```python
from build123d import *

# Parameters (mm, degrees)
SKETCH1_W               = 2.2
SKETCH1_H               = 9.7
SKETCH1_W_2             = 5.7
SKETCH1_H_2             = 3.4
BOSS_EXTRUDE2_DEPTH     = 3
CUT_EXTRUDE2_DEPTH      = 58.983591645
CUT_EXTRUDE2_DEPTH_BACK = 58.983591645
FILLET1_R               = 5
SKETCH4_W               = 20
SKETCH4_H               = 3
BOSS_EXTRUDE3_DEPTH     = 1
SKETCH5_W               = 20
SKETCH5_H               = 1
BOSS_EXTRUDE4_DEPTH     = 10
SKETCH6_W               = 20
SKETCH6_H               = 1.5
BOSS_EXTRUDE5_DEPTH     = 8
SKETCH7_W               = 20
SKETCH7_H               = 3
BOSS_EXTRUDE6_DEPTH     = 1
SKETCH8_W               = 20
SKETCH8_H               = 1
BOSS_EXTRUDE7_DEPTH     = 1.6


with BuildPart() as part:
    # Sketch1 → Boss-Extrude2 (new body)
    with BuildSketch(Plane(origin=(0, 0, 0), x_dir=(1, 0, 0), z_dir=(0, 1, 0))):
        Polygon((0, 15.5), (0, 0), (65, 0), (65, 40), (0, 40), (0, 24.5), (6.46, 24.5), (6.46, 15.5), align=None)
        with Locations((9.45, 20)):
            Rectangle(SKETCH1_W, SKETCH1_H, mode=Mode.SUBTRACT)
        with Locations((55, 20)):
            Rectangle(SKETCH1_W_2, SKETCH1_H_2, mode=Mode.SUBTRACT)
        Polygon((23.13, 11), (23.13, 29), (23.13, 36), (47.2, 36), (47.2, 29), (47.2, 11), (47.2, 4), (23.13, 4), align=None, mode=Mode.SUBTRACT)
    extrude(amount=BOSS_EXTRUDE2_DEPTH)

    # Sketch3 → Cut-Extrude2 (cut, two sides: drawn at the far end of the back side and taken through both)
    with BuildSketch(Plane(origin=(23.13, 0, 0), x_dir=(0, 0, -1), z_dir=(1, 0, 0)).offset(-CUT_EXTRUDE2_DEPTH_BACK)):
        Polygon((11, -0.008080614), (8, 0), (8, 2), (32, 2), (32, 0), align=None)
    extrude(amount=CUT_EXTRUDE2_DEPTH + CUT_EXTRUDE2_DEPTH_BACK, mode=Mode.SUBTRACT)

    # Fillet1
    # the kernel refuses this fillet: 5 mm, written as the material it takes off along each edge
    with BuildSketch(Plane(origin=(57.85, 3, -18.3), x_dir=(0, 0, 1), z_dir=(-1, 0, 0)), Plane(origin=(52.15, 3, -21.7), x_dir=(0, 0, -1), z_dir=(1, 0, 0))) as fillet1_piece_1:
        with BuildLine():
            CenterArc((3, -5), FILLET1_R, 90, 36.869897646)
            Line((0, -1), (0, 0))
            Line((0, 0), (3, 0))
        make_face()
    extrude(amount=5.7, mode=Mode.SUBTRACT)
    with BuildSketch(Plane(origin=(57.85, 3, -21.7), x_dir=(1, 0, 0), z_dir=(0, 0, 1)), Plane(origin=(52.15, 3, -18.3), x_dir=(-1, 0, 0), z_dir=(0, 0, -1))) as fillet1_piece_2:
        with BuildLine():
            CenterArc((3, -5), FILLET1_R, 90, 36.869897646)
            Line((0, -1), (0, 0))
            Line((0, 0), (3, 0))
        make_face()
    extrude(amount=3.4, mode=Mode.SUBTRACT)
    with BuildSketch(Plane(origin=(65.35, 3, -18.3), x_dir=(0, 0, 1), z_dir=(-1, 0, 0))) as fillet1_piece_3a_section:
        with BuildLine():
            CenterArc((3, -5), FILLET1_R, 90, 36.869897646)
            Line((0, -1), (0, 0))
            Line((0, 0), (3, 0))
        make_face()
    fillet1_piece_3a = extrude(amount=13.2, mode=Mode.PRIVATE)
    fillet1_piece_3a = split(fillet1_piece_3a, bisect_by=Plane(origin=(65, 3, -18.3), z_dir=(-1, 0, 0)), keep=Keep.TOP, mode=Mode.PRIVATE)
    fillet1_piece_3a = split(fillet1_piece_3a, bisect_by=Plane(origin=(57.85, 3, -18.3), z_dir=(1, 0, 0)), keep=Keep.TOP, mode=Mode.PRIVATE)
    with BuildSketch(Plane(origin=(57.85, 3, -21.7), x_dir=(1, 0, 0), z_dir=(0, 0, 1))) as fillet1_piece_3b_section:
        with BuildLine():
            CenterArc((3, -5), FILLET1_R, 90, 36.869897646)
            Line((0, -1), (0, 0))
            Line((0, 0), (3, 0))
        make_face()
    fillet1_piece_3b = extrude(amount=10.9, mode=Mode.PRIVATE)
    fillet1_piece_3b = split(fillet1_piece_3b, bisect_by=Plane(origin=(57.85, 3, -18.3), z_dir=(0, 0, 1)), keep=Keep.TOP, mode=Mode.PRIVATE)
    fillet1_piece_3 = fillet1_piece_3a & fillet1_piece_3b
    add(fillet1_piece_3, mode=Mode.SUBTRACT)
    with BuildSketch(Plane(origin=(57.85, 3, -18.3), x_dir=(0, 0, 1), z_dir=(-1, 0, 0))) as fillet1_piece_4a_section:
        with BuildLine():
            CenterArc((3, -5), FILLET1_R, 90, 36.869897646)
            Line((0, -1), (0, 0))
            Line((0, 0), (3, 0))
        make_face()
    fillet1_piece_4a = extrude(amount=13.2, mode=Mode.PRIVATE)
    fillet1_piece_4a = split(fillet1_piece_4a, bisect_by=Plane(origin=(47.2, 3, -18.3), z_dir=(1, 0, 0)), keep=Keep.TOP, mode=Mode.PRIVATE)
    fillet1_piece_4a = split(fillet1_piece_4a, bisect_by=Plane(origin=(52.15, 3, -18.3), z_dir=(-1, 0, 0)), keep=Keep.TOP, mode=Mode.PRIVATE)
    with BuildSketch(Plane(origin=(52.15, 3, -10.8), x_dir=(-1, 0, 0), z_dir=(0, 0, -1))) as fillet1_piece_4b_section:
        with BuildLine():
            CenterArc((3, -5), FILLET1_R, 90, 36.869897646)
            Line((0, -1), (0, 0))
            Line((0, 0), (3, 0))
        make_face()
    fillet1_piece_4b = extrude(amount=10.9, mode=Mode.PRIVATE)
    fillet1_piece_4b = split(fillet1_piece_4b, bisect_by=Plane(origin=(52.15, 3, -18.3), z_dir=(0, 0, 1)), keep=Keep.TOP, mode=Mode.PRIVATE)
    fillet1_piece_4 = fillet1_piece_4a & fillet1_piece_4b
    add(fillet1_piece_4, mode=Mode.SUBTRACT)
    with BuildSketch(Plane(origin=(52.15, 3, -21.7), x_dir=(0, 0, -1), z_dir=(1, 0, 0))) as fillet1_piece_5a_section:
        with BuildLine():
            CenterArc((3, -5), FILLET1_R, 90, 36.869897646)
            Line((0, -1), (0, 0))
            Line((0, 0), (3, 0))
        make_face()
    fillet1_piece_5a = extrude(amount=13.2, mode=Mode.PRIVATE)
    fillet1_piece_5a = split(fillet1_piece_5a, bisect_by=Plane(origin=(65, 3, -21.7), z_dir=(-1, 0, 0)), keep=Keep.TOP, mode=Mode.PRIVATE)
    fillet1_piece_5a = split(fillet1_piece_5a, bisect_by=Plane(origin=(57.85, 3, -21.7), z_dir=(1, 0, 0)), keep=Keep.TOP, mode=Mode.PRIVATE)
    with BuildSketch(Plane(origin=(57.85, 3, -29.2), x_dir=(1, 0, 0), z_dir=(0, 0, 1))) as fillet1_piece_5b_section:
        with BuildLine():
            CenterArc((3, -5), FILLET1_R, 90, 36.869897646)
            Line((0, -1), (0, 0))
            Line((0, 0), (3, 0))
        make_face()
    fillet1_piece_5b = extrude(amount=10.9, mode=Mode.PRIVATE)
    fillet1_piece_5b = split(fillet1_piece_5b, bisect_by=Plane(origin=(57.85, 3, -21.7), z_dir=(0, 0, -1)), keep=Keep.TOP, mode=Mode.PRIVATE)
    fillet1_piece_5 = fillet1_piece_5a & fillet1_piece_5b
    add(fillet1_piece_5, mode=Mode.SUBTRACT)
    with BuildSketch(Plane(origin=(52.15, 3, -18.3), x_dir=(-1, 0, 0), z_dir=(0, 0, -1))) as fillet1_piece_6a_section:
        with BuildLine():
            CenterArc((3, -5), FILLET1_R, 90, 36.869897646)
            Line((0, -1), (0, 0))
            Line((0, 0), (3, 0))
        make_face()
    fillet1_piece_6a = extrude(amount=10.9, mode=Mode.PRIVATE)
    fillet1_piece_6a = split(fillet1_piece_6a, bisect_by=Plane(origin=(52.15, 3, -21.7), z_dir=(0, 0, -1)), keep=Keep.TOP, mode=Mode.PRIVATE)
    with BuildSketch(Plane(origin=(44.65, 3, -21.7), x_dir=(0, 0, -1), z_dir=(1, 0, 0))) as fillet1_piece_6b_section:
        with BuildLine():
            CenterArc((3, -5), FILLET1_R, 90, 36.869897646)
            Line((0, -1), (0, 0))
            Line((0, 0), (3, 0))
        make_face()
    fillet1_piece_6b = extrude(amount=13.2, mode=Mode.PRIVATE)
    fillet1_piece_6b = split(fillet1_piece_6b, bisect_by=Plane(origin=(47.2, 3, -21.7), z_dir=(1, 0, 0)), keep=Keep.TOP, mode=Mode.PRIVATE)
    fillet1_piece_6b = split(fillet1_piece_6b, bisect_by=Plane(origin=(52.15, 3, -21.7), z_dir=(-1, 0, 0)), keep=Keep.TOP, mode=Mode.PRIVATE)
    fillet1_piece_6 = fillet1_piece_6a & fillet1_piece_6b
    add(fillet1_piece_6, mode=Mode.SUBTRACT)

    # Sketch4 → Boss-Extrude3 (add)
    with BuildSketch(Plane(origin=(0, 0, -40), x_dir=(-1, 0, 0), z_dir=(0, 0, -1))):
        with Locations((-10, 1.5)):
            Rectangle(SKETCH4_W, SKETCH4_H)
    extrude(amount=BOSS_EXTRUDE3_DEPTH)

    # Sketch5 → Boss-Extrude4 (add)
    with BuildSketch(Plane.XZ):
        with Locations((10, -40.5)):
            Rectangle(SKETCH5_W, SKETCH5_H)
    extrude(amount=BOSS_EXTRUDE4_DEPTH)

    # Sketch6 → Boss-Extrude5 (add)
    with BuildSketch(Plane.XY.offset(-40)):
        with Locations((10, -9.25)):
            Rectangle(SKETCH6_W, SKETCH6_H)
    extrude(amount=BOSS_EXTRUDE5_DEPTH)

    # Sketch7 → Boss-Extrude6 (add)
    with BuildSketch(Plane.XY):
        with Locations((10, 1.5)):
            Rectangle(SKETCH7_W, SKETCH7_H)
    extrude(amount=BOSS_EXTRUDE6_DEPTH)

    # Sketch8 → Boss-Extrude7 (add)
    with BuildSketch(Plane.XZ):
        with Locations((10, 0.5)):
            Rectangle(SKETCH8_W, SKETCH8_H)
    extrude(amount=BOSS_EXTRUDE7_DEPTH)


solid = part.part
```
Can you work these out from the model? Positions are in its coordinate system, mm. A direction names the side the tool comes from. Coordinates: 2 decimals unless noted, no trailing zeros. Write each loop counter-clockwise with the first axis right and the second up, starting at its lowest first coordinate (ties: lowest second). Pieces come first, ordered by that corner, then holes. Notation, with made-up numbers: M 20.25,27 L 54.25,27 A11 ccw 54.25,40 Z; hole C 12.25,80.25 d5. An arc over 180 degrees is marked long. Answer as CSV lines item,"result".
Item 1: On a 3-axis mill with a long thin cutter (end or side, diameter ignored), from which of +Z, -Z, +X, -X, +Y, -Y can I reach the whole of each face in a straight line? I mean faces 1 (the flat face through (42, 1, 0)), 2 (the flat face through (10, -9, -32)), 3 (the flat face through (10, -1, 0)), 4 (the cylindrical face through (50.37, 2.85, -19.93)), 5 (the flat face through (47.2, 2.5, -20.2)). Say none if no direction works.
Geometry results:
face 1,"+Z, +X, +Y, -Y"
face 2,"+Z, +X, -X, -Y"
face 3,"+X, -X, -Y"
face 4,"+Y"
face 5,"+Y, -Y"
Item 2: We'd pull the mould along Y, two halves only. Please class faces 6 (the flat face through (11, 2, -20)), 7 (the flat face through (10, -4, -40)), 8 (the flat face through (11, 1, -8)): +Y half, -Y half, draft (parallel to the pull), parting line (faces both ways), or undercut.
Geometry results:
face 6,"-Y half"
face 7,"undercut"
face 8,"draft"
Item 3: Imagine slicing it at C-C on z = -19.5. List the corners of the cut face in (x, y) for me, plus the area to 3 significant figures.
Geometry results:
outline,"M 6.46,2 L 8.35,2 L 8.35,3 L 6.46,3 Z; M 10.55,2 L 23.13,2 L 23.13,3 L 10.55,3 Z; M 47.2,2 L 52.15,2 A5 ccw 49.15,3 L 47.2,3 Z; M 57.85,2 L 65,2 L 65,3 L 60.85,3 A5 ccw Z"
area,"24.7 mm2"
Item 4: Imagine slicing it at A-A on z = -9.5. List the corners of the cut face in (x, y) for me, plus the area to 3 significant figures.
Geometry results:
outline,"M 0,2 L 23.13,2 L 23.13,3 L 0,3 Z; M 47.2,2 L 65,2 L 65,3 L 47.2,3 Z"
area,"40.9 mm2"
Item 5: Please list where these lines run through material, in increasing order: line 1 along Z through (x, y) = (47, 0.25); line 2 along Y through (x, z) = (5, -37.5); line 3 along Y through (x, z) = (56.5, -34).
Geometry results:
line 1,"z = -40 to -36, -4 to 0"
line 2,"y = -10 to -8.5, 0 to 3"
line 3,"y = 0 to 3"
Item 6: Imagine slicing it at D-D on z = -33. List the corners of the cut face in (x, y) for me.
Geometry results:
outline,"M 0,-10 L 20,-10 L 20,-8.5 L 0,-8.5 Z; M 0,0 L 23.13,0 L 23.13,3 L 0,3 Z; M 47.2,0 L 65,0 L 65,3 L 47.2,3 Z"
Item 7: I'm going to push flat-ended pins straight in: P1, Ø0.9, axis at y = 1, z = -26.5, coming from the +X side; P2, Ø3.5, axis at x = 30, y = 1.5, coming from the -Z side; P3, Ø3, axis at x = 51.5, z = -15, coming from the -Y side; P4, Ø9, axis at x = 24.5, z = -5, coming from the -Y side. Where does each tip first touch, or does it pass through?
Geometry results:
P1,"passes through"
P2,"stops at z = -40"
P3,"stops at y = 2"
P4,"stops at y = 0"
Item 8: Imagine slicing it at B-B on x = 24. List the corners of the cut face in (y, z) for me, plus the area to 3 significant figures.
Geometry results:
outline,"M 0,-40 L 3,-40 L 3,-36 L 0,-36 Z; M 0,-4 L 3,-4 L 3,0 L 0,0 Z"
area,"24.0 mm2"
